Check sheet for the modelled part. Datum: model origin and axes. Units: mm. Face numbers are marked on the shaded views. A direction names the side the tool comes from. Coordinates: 2 decimals unless noted, no trailing zeros. Loops run counter-clockwise (first coordinate to the right, second up) from the corner with the lowest first, then second, coordinate; pieces in that order, holes last. Notation, with made-up numbers: M 73.25,-36 L 104.25,-36 A19 cw 104.25,-25 Z; hole C 87.5,12.5 d3. An arc over 180 degrees is marked long. Write each question's results on one line, items separated by ' | '. Start each with the question number.
from build123d import *

# Parameters (mm, degrees)
EXTRUDE_1_DEPTH     = 21.5
SKETCH_2_W          = 43.373604633
SKETCH_2_H          = 16.611508938
CUT_EXTRUDE_1_DEPTH = 13.5


with BuildPart() as part:
    # Эскиз1 → Вытянуть1 (new body)
    with BuildSketch(Plane.XY):
        Polygon((-0.0095286, 2), (1.9904714, 0), (29.0095286, 0), (31.0095286, 2), (31.0095286, 10), (36.5, 10), (36.5, 15.9904714), (34.5, 17.9904714), (-3.5, 17.9904714), (-5.5, 15.9904714), (-5.5, 10), (-0.0095286, 10), align=None)
    extrude(amount=EXTRUDE_1_DEPTH)

    # Эскиз2 → Вырез-Вытянуть1 (cut)
    with BuildSketch(Plane(origin=(0, 0, 0), x_dir=(-1, 0, 0), z_dir=(0, 0, -1))):
        with Locations((-15.469303829, 12.305754469)):
            Rectangle(SKETCH_2_W, SKETCH_2_H)
    extrude(amount=-CUT_EXTRUDE_1_DEPTH, mode=Mode.SUBTRACT)


solid = part.part
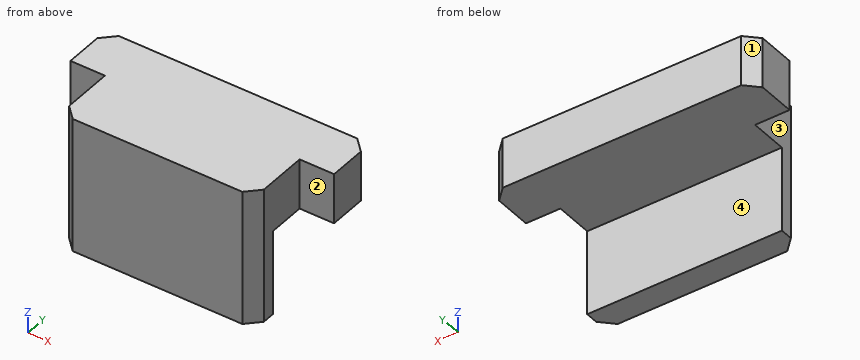
Item 1: Tool access check on the marked faces 1, 2, 3 and 4. Record the directions out of +Z, -Z, +X, -X, +Y, -Y that give a thin tool (end or side, any length) a straight path to the whole face; none if there is none.
Item 2: Thickness scan on line 1 (Z direction, x = 22, y = 10.5); line 2 (Y direction, x = 33.5, z = 15); line 3 (Y direction, x = 13, z = 3.5). Record the ranges inside material, lowest first.
Item 3: Section check C-C (y = 5.75). Record the cut outline in (x, z), plus the area to 3 significant figures.
Item 4: Section check B-B (x = 13.5). Record the cut outline in (y, z).
Item 5: Section check A-A (z = 5.75). Record the cut outline in (x, y).
Item 6: Depth check by flat-ended pin: P1, Ø1.5, axis at x = -0.5, y = 9.5, coming from the -Z side; P2, Ø3, axis at y = 4.5, z = 14, coming from the -X side; P3, Ø2, axis at x = 2, z = 11, coming from the +Y side; P4, Ø5, axis at x = 19.5, z = 16, coming from the -Y side. Enter the tip coordinate at first touch or a pass-through.
Item 7: Section check D-D (y = 12.5). Record the cut outline in (x, z), plus the area to 3 significant figures.
Computed values:
1) face 1: +Z, -Z, -X, +Y | face 2: +Z, -Z, +X, -Y | face 3: +Z, -Z, -X, -Y | face 4: -Z, +X, -X, +Y
2) line 1: z = 13.5 to 21.5 | line 2: y = 10 to 17.99 | line 3: y = 0 to 4
3) outline: M -0.01,13.5 L 31.01,13.5 L 31.01,21.5 L -0.01,21.5 Z | area: 248 mm²
4) outline: M 0,0 L 4,0 L 4,13.5 L 17.99,13.5 L 17.99,21.5 L 0,21.5 Z
5) outline: M -0.01,2 L 1.99,0 L 29.01,0 L 31.01,2 L 31.01,4 L -0.01,4 Z
6) P1: stops at z = 13.5 | P2: stops at x = -0.01 | P3: stops at y = 4 | P4: stops at y = 0
7) outline: M -5.5,13.5 L 36.5,13.5 L 36.5,21.5 L -5.5,21.5 Z | area: 336 mm²
